Could you check a few things on this model? Use its own coordinates, in mm. A direction names the side the tool comes from. Coordinates: 2 decimals unless noted, no trailing zeros. Loops run counter-clockwise (first coordinate to the right, second up) from the corner with the lowest first, then second, coordinate; pieces in that order, holes last. Notation, with made-up numbers: M 53.25,-28.5 L 81.25,-28.5 A12 ccw 81.25,-14.5 Z; hole C 64.25,20 d10. An arc over 180 degrees is marked long. Write each question's results on one line, items separated by ' | '.
```python
from build123d import *

# Parameters (mm, degrees)
BOSS_EXTRUDE1_DEPTH     = 40.2
CUT_EXTRUDE1_DEPTH      = 62.976124435
CUT_EXTRUDE1_DEPTH_BACK = 62.976124435
CUT_EXTRUDE2_DEPTH      = 61.083608414
CUT_EXTRUDE2_DEPTH_BACK = 61.083608414
SKETCH3_R               = 1.35


with BuildPart() as part:
    # Sketch1 → Boss-Extrude1 (new body)
    with BuildSketch(Plane(origin=(0, 0, 0), x_dir=(0, 0, -1), z_dir=(1, 0, 0))):
        Polygon((0, 25), (0, 0), (40, 0), (40, 25), (37, 25), (37, 3), (3, 3), (3, 25), align=None)
    extrude(amount=BOSS_EXTRUDE1_DEPTH)

    # Sketch2 → Cut-Extrude1 (cut, two sides: drawn at the far end of the back side and taken through both)
    with BuildSketch(Plane.XY.offset(-CUT_EXTRUDE1_DEPTH_BACK)):
        with BuildLine():
            Line((20.1, 8.6), (20.1, 25))
            Line((20.1, 25), (5.6, 25))
            Line((5.6, 25), (5.6, 9.6))
            ThreePointArc((5.6, 9.6), (5.892893219, 8.892893219), (6.6, 8.6))
            Line((6.6, 8.6), (20.1, 8.6))
        make_face()
        with BuildLine():
            Line((34.6, 25), (20.1, 25))
            Line((20.1, 25), (20.1, 8.6))
            Line((20.1, 8.6), (33.6, 8.6))
            ThreePointArc((33.6, 8.6), (34.307106781, 8.892893219), (34.6, 9.6))
            Line((34.6, 9.6), (34.6, 25))
        make_face()
    extrude(amount=CUT_EXTRUDE1_DEPTH + CUT_EXTRUDE1_DEPTH_BACK, mode=Mode.SUBTRACT)

    # Sketch3 → Cut-Extrude2 (cut, two sides: drawn at the far end of the back side and taken through both)
    with BuildSketch(Plane(origin=(0, 0, -3), x_dir=(-1, 0, 0), z_dir=(0, 0, -1)).offset(-CUT_EXTRUDE2_DEPTH_BACK)):
        with Locations((-9.1, 5.8)):
            Circle(SKETCH3_R)
        with Locations((-2.8, 11.1)):
            Circle(SKETCH3_R)
        with Locations((-37.4, 11.1)):
            Circle(SKETCH3_R)
        with Locations((-31.1, 5.8)):
            Circle(SKETCH3_R)
    extrude(amount=CUT_EXTRUDE2_DEPTH + CUT_EXTRUDE2_DEPTH_BACK, mode=Mode.SUBTRACT)


solid = part.part
```
(1) Imagine slicing it at C-C, the plane y = 11.1. State how many separate pieces and enclosed holes the cut face has, and give its area (3 significant figures).
Reported:
separate pieces: 8 | enclosed holes: 0 | area: 34.8 mm2
(2) Imagine slicing it at D-D, the plane y = 5.8. List the corners of the cut face in (x, z) for me, and give its area (3 significant figures).
Reported:
outline: M 0,-40 L 7.75,-40 L 7.75,-37 L 0,-37 Z; M 0,-3 L 7.75,-3 L 7.75,0 L 0,0 Z; M 10.45,-40 L 29.75,-40 L 29.75,-37 L 10.45,-37 Z; M 10.45,-3 L 29.75,-3 L 29.75,0 L 10.45,0 Z; M 32.45,-40 L 40.2,-40 L 40.2,-37 L 32.45,-37 Z; M 32.45,-3 L 40.2,-3 L 40.2,0 L 32.45,0 Z | area: 209 mm2
(3) Imagine slicing it at B-B, the plane x = 2.8. List the corners of the cut face in (y, z) for me.
Reported:
outline: M 0,-40 L 9.75,-40 L 9.75,-37 L 3,-37 L 3,-3 L 9.75,-3 L 9.75,0 L 0,0 Z; M 12.45,-40 L 25,-40 L 25,-37 L 12.45,-37 Z; M 12.45,-3 L 25,-3 L 25,0 L 12.45,0 Z
(4) Imagine slicing it at A-A, the plane y = 17.5. List the corners of the cut face in (x, z) for me.
Reported:
outline: M 0,-40 L 5.6,-40 L 5.6,-37 L 0,-37 Z; M 0,-3 L 5.6,-3 L 5.6,0 L 0,0 Z; M 34.6,-40 L 40.2,-40 L 40.2,-37 L 34.6,-37 Z; M 34.6,-3 L 40.2,-3 L 40.2,0 L 34.6,0 Z
(5) Will these pins go through, and if not, where does the flat tip stop? P1, Ø1, axis at x = 7, y = 16, coming from the +Z side; P2, Ø1.5, axis at x = 14.5, z = -26, coming from the +Y side; P3, Ø0.9, axis at x = 24, z = -2, coming from the +Y side.
Reported:
P1: passes through | P2: stops at y = 3 | P3: stops at y = 8.6
(6) If we mould it in two halves opening along X, with no side actions, what happens to faces 1 (the flat face through (20, 7, -3)), 2 (the flat face through (5.6, 17, -39)), 3 (the flat face through (0, 2, -21))? For each: released by +X, released by -X, zero draft, split by the parting line, or undercut.
Reported:
face 1: zero draft | face 2: undercut | face 3: released by -X
(7) Which directions (+Z, -Z, +X, -X, +Y, -Y) give clear straight access to the entire face, cutting with the end or side of a thin tool? Please do faces 4 (the flat face through (37, 25, -2)), 5 (the cylindrical face through (5.885, 8.901, -38.521)).
Reported:
face 4: +Z, -Z, +X, -X, +Y | face 5: +Z, -Z, +Y
(8) Please list where these lines run through material, in increasing order: probe 1 along X at (y, z) = (5.8, -1.35); probe 2 along Y at (x, z) = (9.1, -37.75); probe 3 along X at (y, z) = (11.1, -2.35). Write a range as from..to.
Reported:
probe 1: x = 0..7.75, 10.45..29.75, 32.45..40.2 | probe 2: y = 0..4.45, 7.15..8.6 | probe 3: x = 0..1.45, 4.15..5.6, 34.6..36.05, 38.75..40.2
